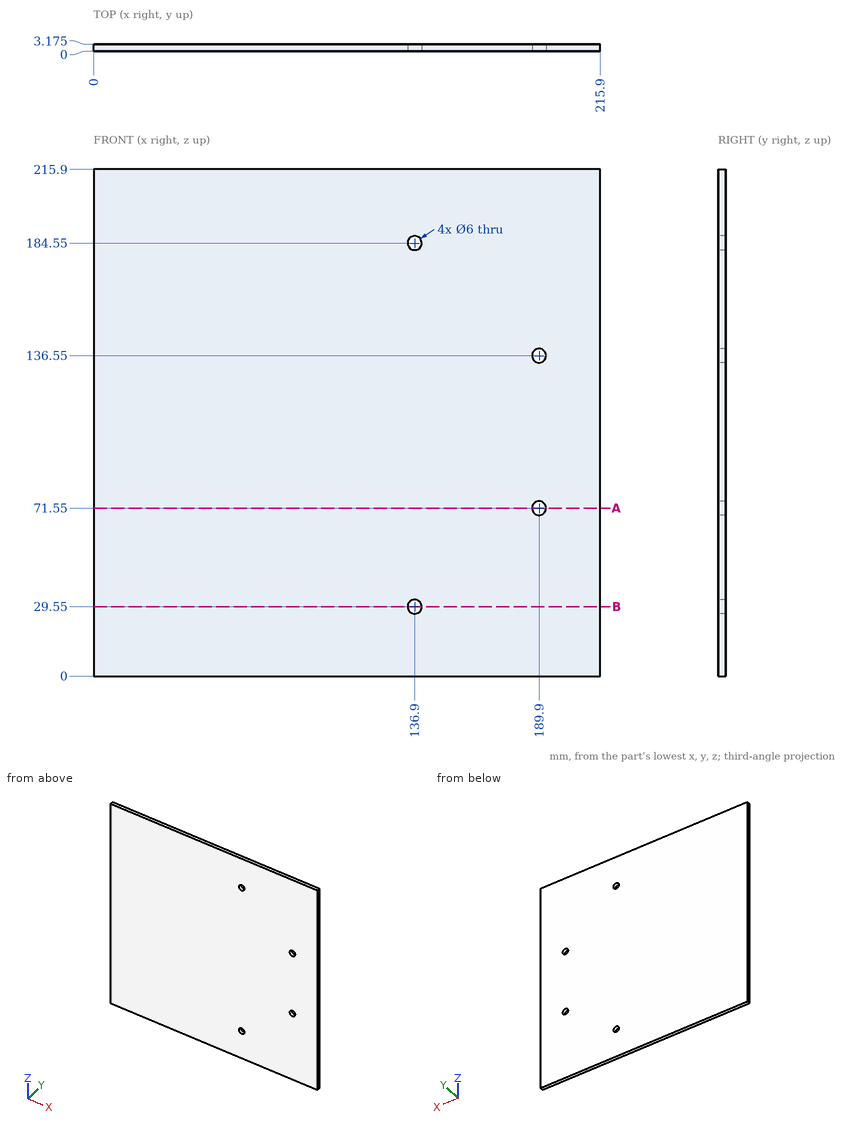
Geometry: see drawing. Coordinates: mm, zero at the bounding-box minimum. Coordinates: 2 decimals unless noted, no trailing zeros. Write each loop counter-clockwise with the first axis right and the second up, starting at its lowest first coordinate (ties: lowest second). Pieces come first, ordered by that corner, then holes. Notation, with made-up numbers: M -36.5,10 L -25.5,10 A25 cw -25.5,26 Z; hole C 13.25,30.25 d3. An arc over 180 degrees is marked long. Answer as a JSON object with one key per item and string values.
1. Ray query, L1, parallel to Z at x = 189.9, y = 2.3; L2, parallel to Z at x = 136.9, y = 2.4; L3, parallel to X at y = 1.75, z = 136.55. Return the intervals inside material, ascending.
Evaluation:
{"L1": "0 to 68.55, 74.55 to 133.55, 139.55 to 215.9", "L2": "0 to 26.55, 32.55 to 181.55, 187.55 to 215.9", "L3": "0 to 186.9, 192.9 to 215.9"}
2. Cut plane B-B on z = 29.55. Output: boundary loops of the cut face in (x, y) (3 decimals).
Evaluation:
{"outline": "M 0,0 L 133.9,0 L 133.9,3.175 L 0,3.175 Z; M 139.9,0 L 215.9,0 L 215.9,3.175 L 139.9,3.175 Z"}
3. Cut plane A-A on z = 71.55. Output: boundary loops of the cut face in (x, y) (3 decimals).
Evaluation:
{"outline": "M 0,0 L 186.9,0 L 186.9,3.175 L 0,3.175 Z; M 192.9,0 L 215.9,0 L 215.9,3.175 L 192.9,3.175 Z"}
